```python
from build123d import *

# Parameters (mm, degrees)
F0_W     = 101
F0_H     = 54
F1_DEPTH = 132.5
F2_T     = -3
F3_W     = 101
F3_H     = 28.575
F4_DEPTH = 3
F6_DEPTH = 3
F7_R     = 1.5


with BuildPart() as f1:
    # F0 (on Top) → F1 (new body, symmetric)
    with BuildSketch(Plane.XY):
        Rectangle(F0_W, F0_H)
    extrude(amount=F1_DEPTH, both=True)

    # F2
    f2_openings = [f1.faces().sort_by_distance(p)[0] for p in [
        (0, 0, 132.5),
    ]]
    offset(amount=F2_T, openings=f2_openings)

    # F3 (on face) → F4 (cut, through all)
    with BuildSketch(Plane.XZ.offset(27)):
        with Locations((0, 118.2125)):
            Rectangle(F3_W, F3_H)
    extrude(amount=-F4_DEPTH, mode=Mode.SUBTRACT)

    # F5 (on face) → F6 (cut, through all)
    with BuildSketch(Plane.XZ.offset(27)):
        with BuildLine():
            Line((-34.29, 94.275), (-34.29, 91.9536233691))
            ThreePointArc((-34.29, 91.9536233691), (-31.75, 83.1625), (-29.21, 91.9536233691))
            Line((-29.21, 91.9536233691), (-29.21, 94.275))
            ThreePointArc((-29.21, 94.275), (-31.75, 96.815), (-34.29, 94.275))
        make_face()
        with BuildLine():
            ThreePointArc((34.29, 94.275), (31.75, 96.815), (29.21, 94.275))
            Line((29.21, 94.275), (29.21, 91.9536233691))
            ThreePointArc((29.21, 91.9536233691), (31.75, 83.1625), (34.29, 91.9536233691))
            Line((34.29, 91.9536233691), (34.29, 94.275))
        make_face()
        with BuildLine():
            Line((-2.54, -54.725), (-2.54, -57.0463766309))
            ThreePointArc((-2.54, -57.0463766309), (0, -65.8375), (2.54, -57.0463766309))
            Line((2.54, -57.0463766309), (2.54, -54.725))
            ThreePointArc((2.54, -54.725), (0, -52.185), (-2.54, -54.725))
        make_face()
    extrude(amount=-F6_DEPTH, mode=Mode.SUBTRACT)

    # F7
    f7_edges = [f1.edges().sort_by_distance(p)[0] for p in [
        (50.5, -27, -14.2875),
        (50.5, 27, 0),
        (-50.5, -27, -14.2875),
        (-50.5, 27, 0),
        (-50.5, 0, -132.5),
        (0, 27, -132.5),
        (0, -27, -132.5),
        (50.5, 0, -132.5),
        (-50.5, 1.5, 132.5),
        (0, 27, 132.5),
        (50.5, 1.5, 132.5),
        (0, -27, 103.925),
        (-50.5, -24, 118.2125),
        (50.5, -24, 118.2125),
    ]]
    fillet(f7_edges, radius=F7_R)


solid = f1.part
```
CAD build for the part. Positions are in the model's coordinates, mm. A direction names the side the tool comes from. Round coordinates to 2 decimals unless told otherwise and drop trailing zeros. Order: outer loops, then holes, each group sorted by start corner. A loop starts at its lowest first (then second) coordinate and runs counter-clockwise, first axis right, second up. Notation, with made-up numbers: (4.5, 22) - (50.5, 22) arc R28 ccw to (50.5, 46) - close; hole circle Ø2 at (47, 88). An arc over 180 degrees is marked (long way). Answer in a Markdown table with one row per item. Add a question column.
(1) Probe L1, parallel to X at y = -14, z = -48.5; L2, parallel to Y at x = -11, z = -81; L3, parallel to Z at x = -41.5, y = -7.5. List the from-to ranges inside material, lowest first. Write a range as [from, to].
(2) Drop flat-ended pins along their axis: pin 1 Ø0.8 at (x, z) = (-48.5, 113) entering from -Y; pin 2 Ø0.7 at (y, z) = (-26, 93.5) entering from -X; pin 3 Ø8.5 at (x, z) = (0, -61.075) entering from -Y; pin 4 Ø15 at (x, z) = (-31.75, 87.925) entering from -Y. Give the stop position or say it passes through.
(3) Band-saw the part on B-B on z = 33.5. List the corners of the cut face in (x, y).
(4) Mould opens along Y. For faces 4 (the face through (-31.922, -25.521, 83.166)), 5 (the face through (-1, -27, -13)), 6 (the face through (-1, 0, -129.5)) say: +Y half, -Y half, draft (parallel to the pull), parting line (faces both ways), or undercut.
(5) Band-saw the part on C-C on x = 14. List the corners of the cut face in (y, z) (3 decimals), and give its area (3 significant figures).
(6) 3-axis set-ups, long thin cutter, end or side, ignore diameter. For faces 1 (the face through (-1, -24, -11)), 2 (the face through (-0.172, -25.521, -65.834)), 3 (the face through (0, 25, 132.5)): which of +Z, -Z, +X, -X, +Y, -Y reach the whole face in a straight line?
(7) Band-saw the part on D-D on y = -15.5. List the corners of the cut face in (x, z).
(8) Band-saw the part on A-A on x = -31.75. List the corners of the cut face in (y, z) (1 decimal).
Data:
| question | item | result |
|---|---|---|
| 1 | L1 | x = [-50.5, -47.5], [47.5, 50.5] |
| 1 | L2 | y = [-27, -24], [24, 27] |
| 1 | L3 | z = [-132.5, -129.5] |
| 2 | pin 1 | stops at y = -24 |
| 2 | pin 2 | stops at x = -50.49 |
| 2 | pin 3 | stops at y = 24 |
| 2 | pin 4 | stops at y = -27 |
| 3 | outline | (-50.5, -25.5) arc R1.5 ccw to (-49, -27) - (49, -27) arc R1.5 ccw to (50.5, -25.5) - (50.5, 25.5) arc R1.5 ccw to (49, 27) - (-49, 27) arc R1.5 ccw to (-50.5, 25.5) - close; hole (-47.5, -24) - (47.5, -24) - (47.5, 24) - (-47.5, 24) - close |
| 4 | face 4 | draft |
| 4 | face 5 | -Y half |
| 4 | face 6 | undercut |
| 5 | outline | (-27, -131) arc R1.5 ccw to (-25.5, -132.5) - (25.5, -132.5) arc R1.5 ccw to (27, -131) - (27, 131) arc R1.5 ccw to (25.5, 132.5) - (24, 132.5) - (24, -129.5) - (-24, -129.5) - (-24, 103.925) - (-25.5, 103.925) arc R1.5 ccw to (-27, 102.425) - close |
| 5 | area | 1,650 mm^2 |
| 6 | face 1 | +Z |
| 6 | face 2 | -Y |
| 6 | face 3 | +Z, +X, -X, +Y, -Y |
| 7 | outline | (-50.5, -131) arc R1.5 ccw to (-49, -132.5) - (49, -132.5) arc R1.5 ccw to (50.5, -131) - (50.5, 131) arc R1.5 ccw to (49, 132.5) - (47.5, 132.5) - (47.5, -129.5) - (-47.5, -129.5) - (-47.5, 132.5) - (-49, 132.5) arc R1.5 ccw to (-50.5, 131) - close |
| 8 | outline | (-27, -131) arc R1.5 ccw to (-25.5, -132.5) - (25.5, -132.5) arc R1.5 ccw to (27, -131) - (27, 131) arc R1.5 ccw to (25.5, 132.5) - (24, 132.5) - (24, -129.5) - (-24, -129.5) - (-24, 83.2) - (-27, 83.2) - close; (-27, 96.8) - (-24, 96.8) - (-24, 103.9) - (-25.5, 103.9) arc R1.5 ccw to (-27, 102.4) - close |
